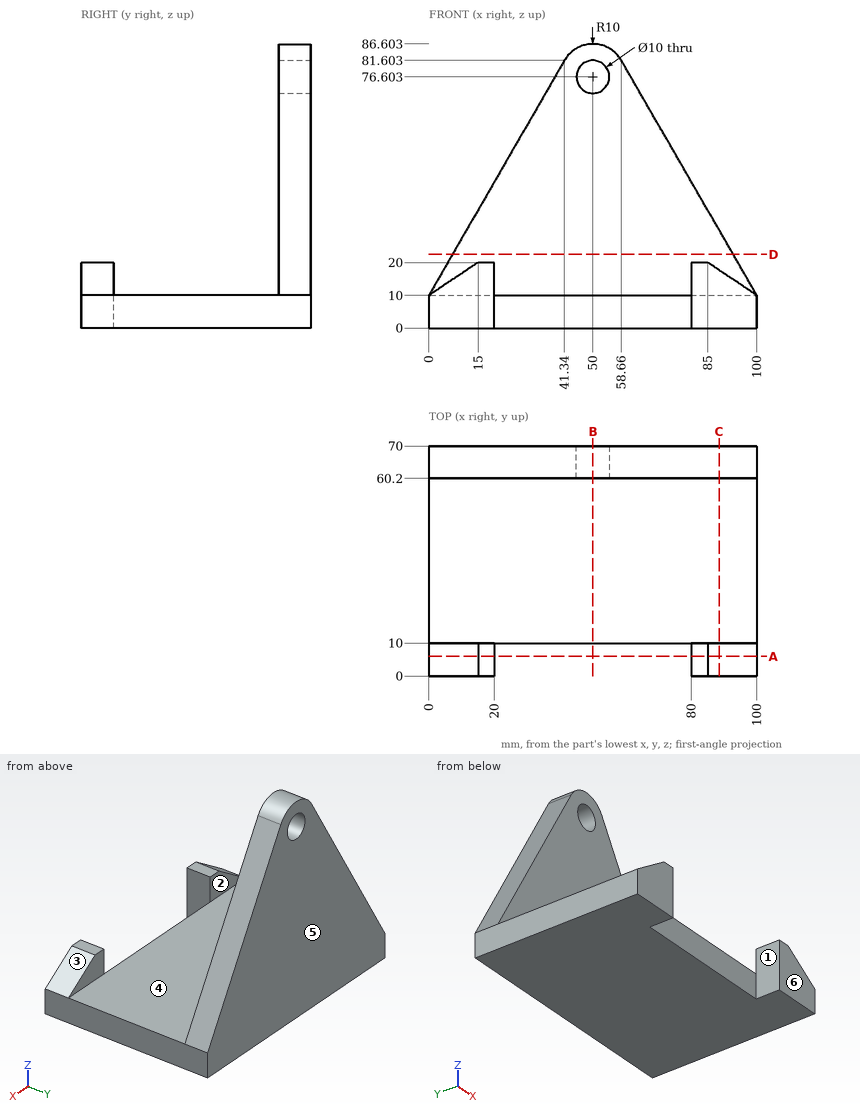
Answer from the drawing. Dimensions are ordinates in mm from the lowest x, y and z of the part. A direction names the side the tool comes from. Round coordinates to 2 decimals unless told otherwise and drop trailing zeros. Loops run counter-clockwise (first coordinate to the right, second up) from the corner with the lowest first, then second, coordinate; pieces in that order, holes last.
Q1. Each of these flat-tipped pins is pushed along its axis until it touches: pin 1 (11 mm diameter, centred on x = 47, z = 5, fed in from -Y); pin 2 (5 mm diameter, centred on x = 50, z = 30.5, fed in from -Y); pin 3 (2.5 mm diameter, centred on x = 81.5, y = 6.5, fed in from +Z). Where does it stop, or does it pass through?
Q2. Section B-B on x = 50 is taken. Write down the section's boundary in (y, z), and give its area (3 significant figures).
Q3. Section D-D on z = 22.5 is taken. Write down the section's boundary in (x, y).
Q4. Section A-A on y = 6 is taken. Write down the section's boundary in (x, z), and give its area (3 significant figures).
Q5. Which of the six approach directions +Z, -Z, +X, -X, +Y, -Y give full straight-line access (tool end or side, diameter ignored) to the marked faces 1, 2 and 3?
Q6. Section C-C on x = 88.5 is taken. Write down the section's boundary in (y, z), and give its area (3 significant figures).
Q7. Consider probe 1 along Y at (x, z) = (9, 12.5); probe 2 along Y at (x, z) = (59, 45); probe 3 along Z at (x, y) = (9, 52). Determine where each line is inside the solid, lowest interval first.
Q8. Determine the mould class of the marked faces 4, 5 and 6 for opening direction Y: released by +Y, released by -Y, zero draft, split by the parting line, or undercut.
Output:
1. pin 1: stops at y = 10
1. pin 2: stops at y = 60.2
1. pin 3: stops at z = 20
2. outline: (10, 0) - (70, 0) - (70, 71.6) - (60.2, 71.6) - (60.2, 10) - (10, 10) - close; (60.2, 81.6) - (70, 81.6) - (70, 86.6) - (60.2, 86.6) - close
2. area: 1,250 mm2
3. outline: (7.22, 60.2) - (92.78, 60.2) - (92.78, 70) - (7.22, 70) - close
4. outline: (0, 0) - (20, 0) - (20, 20) - (15, 20) - (0, 10) - close; (80, 0) - (100, 0) - (100, 10) - (85, 20) - (80, 20) - close
4. area: 650 mm2
5. face 1: +Z, -Z, -Y
5. face 2: +Z, +X, -X
5. face 3: +Z, +X, -Y
6. outline: (0, 0) - (70, 0) - (70, 29.92) - (60.2, 29.92) - (60.2, 10) - (10, 10) - (10, 17.67) - (0, 17.67) - close
6. area: 972 mm2
7. probe 1: y = 0 to 10, 60.2 to 70
7. probe 2: y = 60.2 to 70
7. probe 3: z = 0 to 10
8. face 4: undercut
8. face 5: released by +Y
8. face 6: released by -Y
